```python
from build123d import *

# Parameters (mm, degrees)
SKETCH_1_W         = 33
SKETCH_1_H         = 30
SKETCH_1_R         = 1.6
EXTRUDE_1_DEPTH    = 4
SKETCH2_W          = 17
SKETCH2_H          = 5
CUT_EXTRUDE2_DEPTH = 5


with BuildPart() as part:
    # Эскиз1 → Бобышка-Вытянуть1 (new body)
    with BuildSketch(Plane(origin=(15.473923778, 0, 0), x_dir=(0, 0, -1), z_dir=(1, 0, 0))):
        with Locations((3.263696673, 23.493617857)):
            Rectangle(SKETCH_1_W, SKETCH_1_H)
        with Locations((-7.236303327, 31.493617857)):
            Circle(SKETCH_1_R, mode=Mode.SUBTRACT)
        with Locations((12.763696673, 31.493617857)):
            Circle(SKETCH_1_R, mode=Mode.SUBTRACT)
        with Locations((-7.236303327, 15.493617857)):
            Circle(SKETCH_1_R, mode=Mode.SUBTRACT)
        with Locations((12.763696673, 15.493617857)):
            Circle(SKETCH_1_R, mode=Mode.SUBTRACT)
    extrude(amount=EXTRUDE_1_DEPTH)

    # Sketch2 → Cut-Extrude2 (cut, through all)
    with BuildSketch(Plane.ZY.offset(-15.473923778)):
        with Locations((-2.763696673, 23.493617857)):
            Rectangle(SKETCH2_W, SKETCH2_H)
    extrude(amount=-CUT_EXTRUDE2_DEPTH, mode=Mode.SUBTRACT)


solid = part.part
```
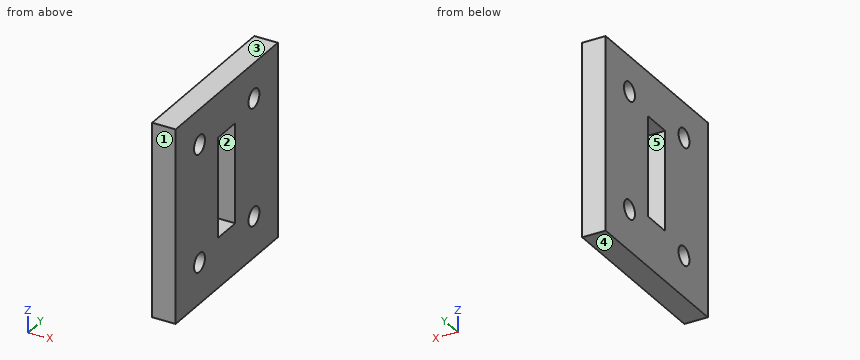
Here's how the part is built. I have some questions about the finished solid (model axes, mm). Face numbers are marked on the shaded views. A direction names the side the tool comes from. Round coordinates to 2 decimals unless told otherwise and drop trailing zeros. Order: outer loops, then holes, each group sorted by start corner. A loop starts at its lowest first (then second) coordinate and runs counter-clockwise, first axis right, second up. Notation, with made-up numbers: M -20,1.25 L -10,1.25 A13 ccw -10,6.25 Z; hole C 84,-33 d1. An arc over 180 degrees is marked long. Answer in a Markdown table with one row per item.
Item 1: If I drill on L1, parallel to Y at x = 16.25, z = -1; L2, parallel to Z at x = 15.7, y = 24.5; L3, parallel to Y at x = 16.4, z = 6, over which ranges is the centre line in solid material (lowest first)? Write a range as from..to.
A:
| item | result |
|---|---|
| L1 | y = 8.49..20.99, 25.99..38.49 |
| L2 | z = -19.76..-11.26, 5.74..13.24 |
| L3 | y = 8.49..14.48, 16.51..30.48, 32.51..38.49 |
Item 2: Imagine slicing it at A-A, the plane z = 0. Write out the boundary of the cut face in (x, y), and give its area (3 significant figures).
A:
| item | result |
|---|---|
| outline | M 15.47,8.49 L 19.47,8.49 L 19.47,20.99 L 15.47,20.99 Z; M 15.47,25.99 L 19.47,25.99 L 19.47,38.49 L 15.47,38.49 Z |
| area | 100 mm2 |
Item 3: Imagine slicing it at B-B, the plane y = 14.5. Write out the boundary of the cut face in (x, z).
A:
| item | result |
|---|---|
| outline | M 15.47,-19.76 L 19.47,-19.76 L 19.47,-14.02 L 15.47,-14.02 Z; M 15.47,-11.51 L 19.47,-11.51 L 19.47,5.98 L 15.47,5.98 Z; M 15.47,8.49 L 19.47,8.49 L 19.47,13.24 L 15.47,13.24 Z |
Item 4: I'm going to push a flat-ended pin straight in: pin 1 (3.5 mm diameter, centred on y = 31.49, z = -12.76, fed in from +X). Where does the tip first touch, or does it pass through?
A:
| item | result |
|---|---|
| pin 1 | stops at x = 19.47 |
Item 5: Imagine slicing it at C-C, the plane x = 19. Write out the boundary of the cut face in (y, z).
A:
| item | result |
|---|---|
| outline | M 8.49,-19.76 L 38.49,-19.76 L 38.49,13.24 L 8.49,13.24 Z; hole C 15.49,-12.76 d3.2; hole C 15.49,7.24 d3.2; hole M 20.99,-11.26 L 25.99,-11.26 L 25.99,5.74 L 20.99,5.74 Z; hole C 31.49,-12.76 d3.2; hole C 31.49,7.24 d3.2 |
Item 6: For the marked faces 4 and 5, which set-ups out of +Z, -Z, +X, -X, +Y, -Y let a thin tool reach every point of the face, with its end or its side?
A:
| item | result |
|---|---|
| face 4 | -Z, +X, -X, +Y, -Y |
| face 5 | +X, -X |
Item 7: Thinking about a two-plate mould opening in Y: for the marked faces 1, 2 and 3, which applies, +Y half, -Y half, draft (parallel to the pull), parting line (faces both ways), or undercut?
A:
| item | result |
|---|---|
| face 1 | -Y half |
| face 2 | undercut |
| face 3 | draft |
